Check sheet for the modelled part. Datum: model origin and axes. Units: mm. A direction names the side the tool comes from. Give positions to 0.01 mm unless a question says otherwise; leave off trailing zeros. Write each loop counter-clockwise with the first axis right and the second up, starting at its lowest first coordinate (ties: lowest second). Pieces come first, ordered by that corner, then holes. Notation, with made-up numbers: (58.25, 28) -> (69.25, 28) arc R20 ccw to (69.25, 60) -> close; hole circle Ø11 at (61, 64.5). An arc over 180 degrees is marked (long way). Write each question's results on one line, items separated by ' | '. Start each with the question number.
```python
from build123d import *

# Parameters (mm, degrees)
F1_DEPTH = 70
F3_DEPTH = 68
F4_R     = 1


with BuildPart() as f1:
    # F0 (on Top) → F1 (new body)
    with BuildSketch(Plane.XY):
        Polygon((20.09286, -24.115758), (31.260213, -2.844618), (24.115758, 20.09286), (2.844618, 31.260213), (-20.09286, 24.115758), (-31.260213, 2.844618), (-24.115758, -20.09286), (-2.844618, -31.260213), align=None)
    extrude(amount=F1_DEPTH)

    # F2 (on face) → F3 (cut)
    with BuildSketch(Plane.XY.offset(70)):
        Polygon((18.360717, -22.036813), (28.565367, -2.599392), (22.036813, 18.360717), (2.599392, 28.565367), (-18.360717, 22.036813), (-28.565367, 2.599392), (-22.036813, -18.360717), (-2.599392, -28.565367), align=None)
    extrude(amount=-F3_DEPTH, mode=Mode.SUBTRACT)

    # F4
    f4_edges = [f1.edges().sort_by_distance(p)[0] for p in [
        (25.676537, -13.480188, 70),
        (27.687985, 8.624121, 70),
        (13.480188, 25.676537, 70),
        (-8.624121, 27.687985, 70),
        (-25.676537, 13.480188, 70),
        (-27.687985, -8.624121, 70),
        (-13.480188, -25.676537, 70),
        (8.624121, -27.687985, 70),
    ]]
    fillet(f4_edges, radius=F4_R)


solid = f1.part
```
Item 1: Set-up check for faces 1 (the cylindrical face through (-13.2, -25.5, 69.7)), 2 (the flat face through (12.454, 23.392, 36.476)): record each of +Z, -Z, +X, -X, +Y, -Y from which the full face is reachable in a straight line by a thin tool's end or side.
Item 2: Depth check by flat-ended pin: pin 1 Ø6 at (y, z) = (-23.5, 34) entering from -X; pin 2 Ø8 at (x, z) = (1, 19.5) entering from +Y; pin 3 Ø3 at (y, z) = (-19.5, 59.5) entering from -X. Enter the tip coordinate at first touch or a pass-through.
Item 3: Section check A-A on z = 8. Record the boundary of the cut face in (x, y).
Item 4: Mould release check, pull along X, two halves, no side actions. Record for faces 3 (the flat face through (7.73, -25.35, 36.48)), 4 (the flat face through (27.74, 8.46, 34.02)), 5 (the cylindrical face through (-25.5, 13.2, 69.7)): pulls with the +X half, pulls with the -X half, needs draft (parallel to the pull), parting line crosses it, or undercut.
Item 5: Thickness scan on probe 1 along Z at (x, y) = (-4.5, 1.5); probe 2 along Y at (x, z) = (19, 15); probe 3 along X at (y, z) = (11, 14.5). Record the ranges inside material, lowest first. Write a range as from..to.
Check sheet entries:
1) face 1: +Z, -X, -Y | face 2: +Z
2) pin 1: stops at x = -23.34 | pin 2: stops at y = 31.26 | pin 3: stops at x = -24.77
3) outline: (-31.26, 2.84) -> (-24.12, -20.09) -> (-2.84, -31.26) -> (20.09, -24.12) -> (31.26, -2.84) -> (24.12, 20.09) -> (2.84, 31.26) -> (-20.09, 24.12) -> close; hole (-28.57, 2.6) -> (-22.04, -18.36) -> (-2.6, -28.57) -> (18.36, -22.04) -> (28.57, -2.6) -> (22.04, 18.36) -> (2.6, 28.57) -> (-18.36, 22.04) -> close
4) face 3: undercut | face 4: pulls with the +X half | face 5: pulls with the -X half
5) probe 1: z = 0..2 | probe 2: y = -24.46..-20.82, 19.96..22.78 | probe 3: x = -26.98..-24.16, 24.33..26.95
